Part model, mm, in its own coordinate system. Face numbers are marked on the shaded views. Give positions to 0.01 mm unless a question says otherwise; leave off trailing zeros. Order: outer loops, then holes, each group sorted by start corner. A loop starts at its lowest first (then second) coordinate and runs counter-clockwise, first axis right, second up. Notation, with made-up numbers: M -4.75,11 L 51.25,11 A13 ccw 51.25,33 Z; hole C 18,-24 d11. An arc over 180 degrees is marked long. Return JSON: item names as keys, results as strings.
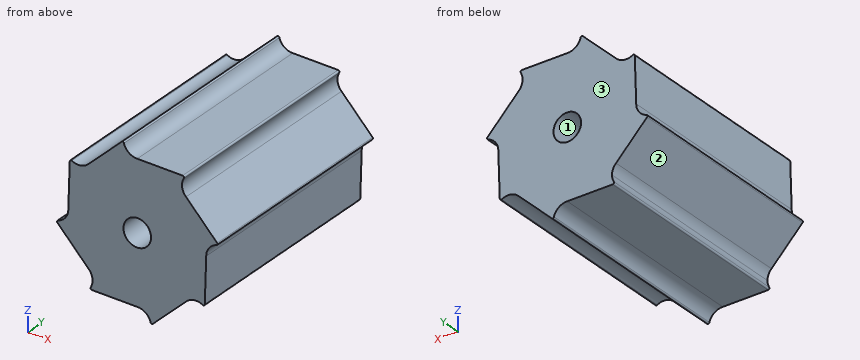
from build123d import *

# Parameters (mm, degrees)
F1_DEPTH = 203.2
F2_R     = 12.7
F3_DEPTH = 203.201
F4_R     = 1.27


with BuildPart() as f1:
    # F0 (on Front) → F1 (new body)
    with BuildSketch(Plane.XZ):
        with BuildLine():
            Line((44.901281, -44.901281), (0, 0))
            Line((0, 0), (-44.901281, -44.901281))
            ThreePointArc((-44.901281, -44.901281), (-42.148267, -49.021457), (-41.181537, -53.881537))
            ThreePointArc((-41.181537, -53.881537), (-41.955794, -58.248076), (-44.184162, -62.082202))
            Line((-44.184162, -62.082202), (0, -63.5))
            ThreePointArc((0, -63.5), (8.597941, -66.853053), (12.655826, -75.141667))
            Line((12.655826, -75.141667), (44.901281, -44.901281))
        make_face()
        with BuildLine():
            ThreePointArc((63.5, 0), (66.853053, 8.597941), (75.141667, 12.655826))
            Line((75.141667, 12.655826), (44.901281, 44.901281))
            Line((44.901281, 44.901281), (0, 0))
            Line((0, 0), (44.901281, -44.901281))
            ThreePointArc((44.901281, -44.901281), (53.351909, -41.192585), (62.082202, -44.184162))
            Line((62.082202, -44.184162), (63.5, 0))
        make_face()
        with BuildLine():
            Line((0, 0), (44.901281, 44.901281))
            ThreePointArc((44.901281, 44.901281), (41.192585, 53.351909), (44.184162, 62.082202))
            Line((44.184162, 62.082202), (0, 63.5))
            ThreePointArc((0, 63.5), (-8.597941, 66.853053), (-12.655826, 75.141667))
            Line((-12.655826, 75.141667), (-44.901281, 44.901281))
            Line((-44.901281, 44.901281), (0, 0))
        make_face()
        with BuildLine():
            Line((-44.901281, -44.901281), (0, 0))
            Line((0, 0), (-44.901281, 44.901281))
            ThreePointArc((-44.901281, 44.901281), (-53.351909, 41.192585), (-62.082202, 44.184162))
            Line((-62.082202, 44.184162), (-63.5, 0))
            ThreePointArc((-63.5, 0), (-66.853053, -8.597941), (-75.141667, -12.655826))
            Line((-75.141667, -12.655826), (-44.901281, -44.901281))
        make_face()
    extrude(amount=F1_DEPTH)

    # F2 (on face) → F3 (cut, through all)
    with BuildSketch(Plane.XZ.offset(203.2)):
        Circle(F2_R)
    extrude(amount=-F3_DEPTH, mode=Mode.SUBTRACT)

    # F4
    f4_edges = [f1.edges().sort_by_distance(p)[0] for p in [
        (-12.655826, -101.6, 75.141667),
        (44.184162, -101.6, 62.082202),
        (-62.082202, -101.6, 44.184162),
        (-75.141667, -101.6, -12.655826),
        (-44.184162, -101.6, -62.082202),
        (12.655826, -101.6, -75.141667),
        (62.082202, -101.6, -44.184162),
        (75.141667, -101.6, 12.655826),
    ]]
    fillet(f4_edges, radius=F4_R)


solid = f1.part
Q1. Band-saw the part on D-D (x = -21). Give the cut face in (y, z), then the cut area to 3 significant figures.
Established:
{"outline": "M -203.2,-62.83 L 0,-62.83 L 0,67.32 L -203.2,67.32 Z", "area": "26,400 mm²"}
Q2. Band-saw the part on A-A (y = -169). Give the cut face in (x, z).
Established:
{"outline": "M -73.53,-14.37 L -44.9,-44.9 A12.7 cw -41.18,-53.88 A12.7 cw -42.89,-60.25 A1.27 ccw -41.84,-62.16 L 0,-63.5 A12.7 cw 12.27,-72.93 A1.27 ccw 14.37,-73.53 L 44.9,-44.9 A12.7 cw 60.25,-42.89 A1.27 ccw 62.16,-41.84 L 63.5,0 A12.7 cw 72.93,12.27 A1.27 ccw 73.53,14.37 L 44.9,44.9 A12.7 cw 42.89,60.25 A1.27 ccw 41.84,62.16 L 0,63.5 A12.7 cw -12.27,72.93 A1.27 ccw -14.37,73.53 L -44.9,44.9 A12.7 cw -60.25,42.89 A1.27 ccw -62.16,41.84 L -63.5,0 A12.7 cw -72.93,-12.27 A1.27 ccw Z; hole C 0,0 d25.4"}
Q3. Two-plate mould, pull along Z, no slides. Class the marked faces 1, 2 and 3: +Z half, -Z half, draft (parallel to the pull), parting line (faces both ways), or undercut.
Established:
{"face 1": "undercut", "face 2": "-Z half", "face 3": "draft"}
Q4. Probe line 1 along Z through (x, y) = (0, -91); line 2 along X through (y, z) = (-30, 9); line 3 along X through (y, z) = (-134.5, 3). List the from-to ranges inside material, lowest first.
Established:
{"line 1": "z = -63.5 to -12.7, 12.7 to 63.5", "line 2": "x = -63.21 to -8.96, 8.96 to 67.24", "line 3": "x = -63.4 to -12.34, 12.34 to 63.86"}
Q5. Band-saw the part on B-B (z = -7.5). Give the cut face in (x, y), then the cut area to 3 significant figures.
Established:
{"outline": "M -65.95,-203.2 L -10.25,-203.2 L -10.25,0 L -65.95,0 Z; M 10.25,-203.2 L 63.26,-203.2 L 63.26,0 L 10.25,0 Z", "area": "22,100 mm²"}
Q6. Band-saw the part on C-C (x = 32). Give the cut face in (y, z), then the cut area to 3 significant figures.
Established:
{"outline": "M -203.2,-57 L 0,-57 L 0,62.47 L -203.2,62.47 Z", "area": "24,300 mm²"}
Q7. Pin check, flat tips, straight feed: pin 1 (4 mm diameter, centred on y = -147, z = -52.5, fed in from +X); pin 2 (8 mm diameter, centred on x = -14, y = -57, fed in from -Z); pin 3 (8 mm diameter, centred on x = 25.5, y = -69, fed in from +Z); pin 4 (5 mm diameter, centred on x = -10, z = 18.5, fed in from +Y). Stop position of each tip, or through.
Established:
{"pin 1": "stops at x = 38.93", "pin 2": "stops at z = -63.18", "pin 3": "stops at z = 62.81", "pin 4": "stops at y = 0"}
